Geometry check sheet. Reference: drawing and pictorial views, mm from the part's lowest x, y, z. A direction names the side the tool comes from. Coordinates: 2 decimals unless noted, no trailing zeros. Write each loop counter-clockwise with the first axis right and the second up, starting at its lowest first coordinate (ties: lowest second). Pieces come first, ordered by that corner, then holes. Notation, with made-up numbers: (51.5, 16) -> (81.5, 16) arc R22 ccw to (81.5, 40) -> close; hole circle Ø9 at (12, 85.5). An arc over 180 degrees is marked (long way). Use a Markdown table: item, result. Add a question column.
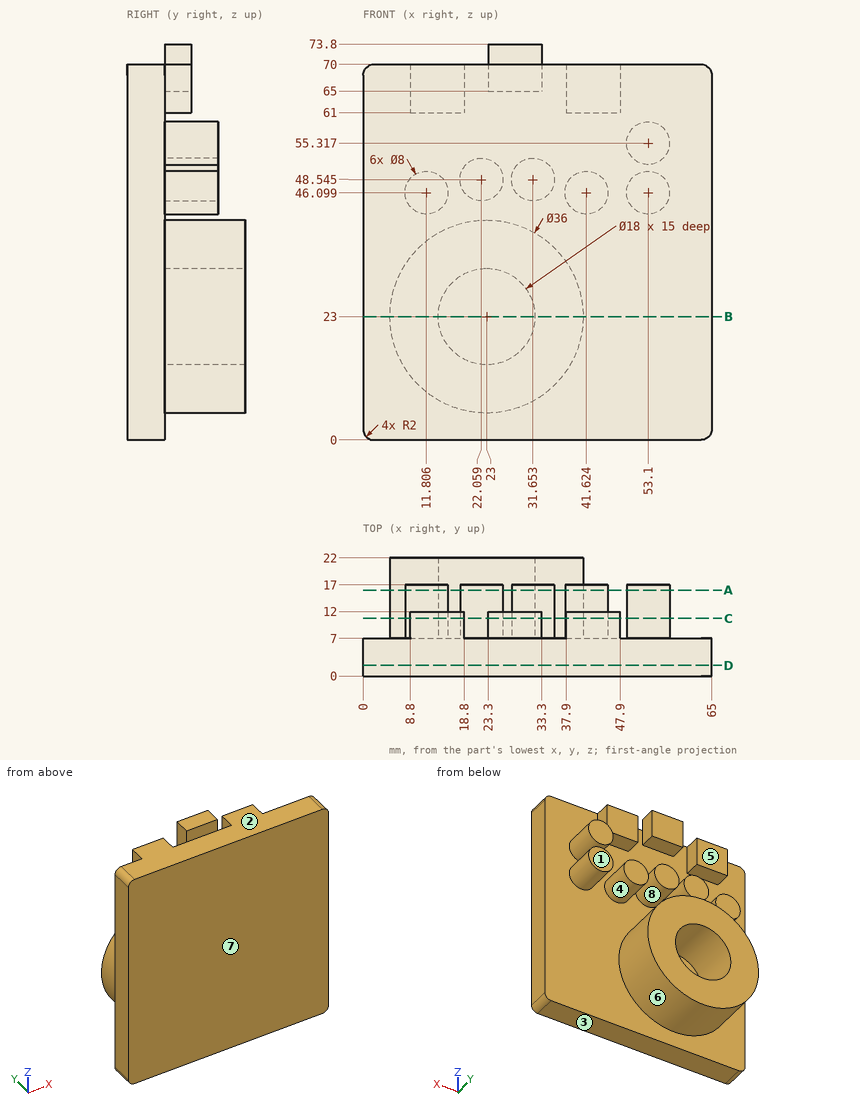
1) Cross-section at A-A on y = 16. Record the boundary of the cut face in (x, z) (1 decimal), then the cut area to 4 significant figures.
2) Release check for a two-part mould opening along X. For the marked faces 6, 7 and 8 record: released by +X, released by -X, zero draft, split by the parting line, or undercut.
3) Gauge pin test, flat ends, axial feed: pin 1 (2.5 mm diameter, centred on y = 8.5, z = 65.5, fed in from -X); pin 2 (9 mm diameter, centred on x = 41, z = 44.5, fed in from +Y); pin 3 (4.5 mm diameter, centred on x = 26, z = 69.5, fed in from +Y). Record the tip position at first contact, or that the pin passes through.
4) Set-up check for the marked faces 1, 2, 3, 4 and 5: record each of +Z, -Z, +X, -X, +Y, -Y from which the full face is reachable in a straight line by a thin tool's end or side.
5) Cross-section at B-B on z = 23. Record the boundary of the cut face in (x, y).
6) Thickness scan on L1, parallel to X at y = 11.25, z = 23; L2, parallel to Z at x = 53, y = 12.25; L3, parallel to Y at x = 14, z = 57.5. Record the ranges inside material, lowest first.
7) Cross-section at C-C on y = 10.75. Give the number of separate pieces and of enclosed holes in the cut face, then the cut area to 3 significant figures.
8) Cross-section at D-D on y = 2. Record the boundary of the cut face in (x, z), then the cut area to 3 significant figures.
Returned:
| question | item | result |
|---|---|---|
| 1 | outline | circle Ø36 at (23, 23); circle Ø8 at (11.8, 46.1); circle Ø8 at (22.1, 48.5); circle Ø8 at (31.7, 48.5); circle Ø8 at (41.6, 46.1); circle Ø8 at (53.1, 46.1); circle Ø8 at (53.1, 55.3); hole circle Ø18 at (23, 23) |
| 1 | area | 1,065 mm² |
| 2 | face 6 | split by the parting line |
| 2 | face 7 | zero draft |
| 2 | face 8 | undercut |
| 3 | pin 1 | stops at x = 8.8 |
| 3 | pin 2 | stops at y = 17 |
| 3 | pin 3 | stops at y = 12 |
| 4 | face 1 | +Z, -Z, +X, -X, +Y |
| 4 | face 2 | +Z, -Y |
| 4 | face 3 | -Z, +X, -X, +Y, -Y |
| 4 | face 4 | +Y |
| 4 | face 5 | +Z, +X, -X, +Y |
| 5 | outline | (0, 0) -> (65, 0) -> (65, 7) -> (41, 7) -> (41, 22) -> (32, 22) -> (32, 7) -> (14, 7) -> (14, 22) -> (5, 22) -> (5, 7) -> (0, 7) -> close |
| 6 | L1 | x = 5 to 14, 32 to 41 |
| 6 | L2 | z = 42.1 to 50.1, 51.32 to 59.32 |
| 6 | L3 | y = 0 to 7 |
| 7 | separate pieces | 10 |
| 7 | enclosed holes | 1 |
| 7 | area | 1,330 mm² |
| 8 | outline | (0, 2) arc R2 ccw to (2, 0) -> (63, 0) arc R2 ccw to (65, 2) -> (65, 68) arc R2 ccw to (63, 70) -> (2, 70) arc R2 ccw to (0, 68) -> close |
| 8 | area | 4,550 mm² |
